The listing builds one solid part. Answer for the finished solid, in the listing's coordinates (mm). Face numbers are marked on the shaded views. A direction names the side the tool comes from. Coordinates: 2 decimals unless noted, no trailing zeros. Write each loop counter-clockwise with the first axis right and the second up, starting at its lowest first coordinate (ties: lowest second). Pieces come first, ordered by that corner, then holes. Notation, with made-up numbers: M 25.5,58 L 77.5,58 A19 ccw 77.5,63 Z; hole C 42,56.5 d7. An arc over 180 degrees is marked long. Answer as a JSON object with one key per item and string values. Group by question number.
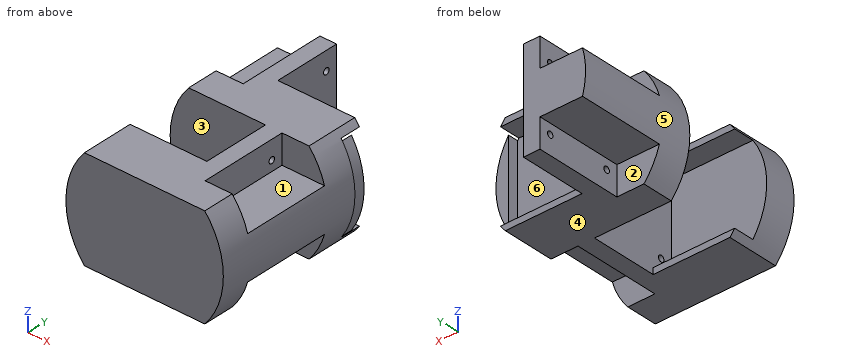
from build123d import *

# Parameters (mm, degrees)
SKETCH1_W           = 76
SKETCH1_H           = 43
BOSS_EXTRUDE1_DEPTH = 15
SKETCH3_W           = 30
SKETCH3_H           = 43
BOSS_EXTRUDE2_DEPTH = 42.1
BOSS_EXTRUDE3_START = 42.1
SKETCH4_W           = 76
SKETCH4_H           = 43
BOSS_EXTRUDE3_DEPTH = 15
SKETCH5_W           = 30
SKETCH5_H           = 43
BOSS_EXTRUDE4_DEPTH = 42.1
BOSS_EXTRUDE5_DEPTH = 3
BOSS_EXTRUDE6_DEPTH = 3
SKETCH2_OUTSIDE_W   = 107.134
SKETCH2_OUTSIDE_H   = 80.134
SKETCH2_OUTSIDE_R   = 38
CUT_EXTRUDE1_DEPTH  = 123.82463108
BOSS_EXTRUDE7_DEPTH = 5
CUT_EXTRUDE2_START  = 16
SKETCH9_W           = 14
SKETCH9_H           = 42.1
CUT_EXTRUDE2_DEPTH  = 40
CUT_EXTRUDE3_START  = -8
SKETCH10_W          = 14
SKETCH10_H          = 42.1
CUT_EXTRUDE3_DEPTH  = 40
SKETCH11_R          = 1.5
CUT_EXTRUDE4_DEPTH  = 60


with BuildPart() as part:
    # Sketch1 → Boss-Extrude1 (new body)
    with BuildSketch(Plane(origin=(0, 0, 0), x_dir=(1, 0, 0), z_dir=(0, 1, 0))):
        Rectangle(SKETCH1_W, SKETCH1_H)
    extrude(amount=BOSS_EXTRUDE1_DEPTH)

    # Sketch3 → Boss-Extrude2 (add)
    with BuildSketch(Plane(origin=(0, 15, 0), x_dir=(1, 0, 0), z_dir=(0, 1, 0))):
        with Locations((23, 0)):
            Rectangle(SKETCH3_W, SKETCH3_H)
    extrude(amount=BOSS_EXTRUDE2_DEPTH)

    # Sketch4 → Boss-Extrude3 (add)
    with BuildSketch(Plane(origin=(0, 15, 0), x_dir=(1, 0, 0), z_dir=(0, 1, 0)).offset(BOSS_EXTRUDE3_START)):
        Rectangle(SKETCH4_W, SKETCH4_H)
    extrude(amount=BOSS_EXTRUDE3_DEPTH)

    # Sketch5 → Boss-Extrude4 (add)
    with BuildSketch(Plane(origin=(0, 72.1, 0), x_dir=(1, 0, 0), z_dir=(0, 1, 0))):
        with Locations((-23, 0)):
            Rectangle(SKETCH5_W, SKETCH5_H)
    extrude(amount=BOSS_EXTRUDE4_DEPTH)

    # Sketch6 → Boss-Extrude5 (add)
    with BuildSketch(Plane.XY.offset(21.5)):
        Polygon((-38, 0), (38, 0), (38, 82.1), (-8, 82.1), (-8, 114.2), (-38, 114.2), (-38, 57.1), (8, 57.1), (8, 25), (-38, 25), align=None)
    extrude(amount=BOSS_EXTRUDE5_DEPTH)

    # Sketch7 → Boss-Extrude6 (add)
    with BuildSketch(Plane(origin=(0, 0, -21.5), x_dir=(-1, 0, 0), z_dir=(0, 0, -1))):
        Polygon((-38, 0), (38, 0), (38, 15), (38, 25), (-8, 25), (-8, 57.1), (38, 57.1), (38, 114.2), (8, 114.2), (8, 82.1), (-38, 82.1), (-38, 72.1), align=None)
    extrude(amount=BOSS_EXTRUDE6_DEPTH)

    # Sketch2 outside → Cut-Extrude1 (cut, through all)
    with BuildSketch(Plane(origin=(0, 0, 0), x_dir=(1, 0, 0), z_dir=(0, 1, 0))):
        Rectangle(SKETCH2_OUTSIDE_W, SKETCH2_OUTSIDE_H)
        Circle(SKETCH2_OUTSIDE_R, mode=Mode.SUBTRACT)
    extrude(amount=CUT_EXTRUDE1_DEPTH, mode=Mode.SUBTRACT)

    # Sketch8 → Boss-Extrude7 (add)
    with BuildSketch(Plane(origin=(0, 72.1, 0), x_dir=(1, 0, 0), z_dir=(0, 1, 0))):
        with BuildLine():
            Line((31.9, -20.64921306), (31.9, 20.64921306))
            ThreePointArc((31.9, 20.64921306), (38, 0), (31.9, -20.64921306))
        make_face()
    extrude(amount=BOSS_EXTRUDE7_DEPTH)

    # Sketch9 → Cut-Extrude2 (cut)
    with BuildSketch(Plane(origin=(0, 0, 0), x_dir=(0, 0, -1), z_dir=(1, 0, 0)).offset(CUT_EXTRUDE2_START)):
        with Locations((-17.5, 36.05)):
            Rectangle(SKETCH9_W, SKETCH9_H)
        with Locations((17.5, 36.05)):
            Rectangle(SKETCH9_W, SKETCH9_H)
    extrude(amount=CUT_EXTRUDE2_DEPTH, mode=Mode.SUBTRACT)

    # Sketch10 → Cut-Extrude3 (cut)
    with BuildSketch(Plane(origin=(-8, 0, 0), x_dir=(0, 0, -1), z_dir=(1, 0, 0)).offset(CUT_EXTRUDE3_START)):
        with Locations((-17.5, 93.15)):
            Rectangle(SKETCH10_W, SKETCH10_H)
        with Locations((17.5, 93.15)):
            Rectangle(SKETCH10_W, SKETCH10_H)
    extrude(amount=-CUT_EXTRUDE3_DEPTH, mode=Mode.SUBTRACT)

    # Sketch11 → Cut-Extrude4 (cut)
    with BuildSketch(Plane(origin=(16, 0, 0), x_dir=(0, 0, -1), z_dir=(1, 0, 0))):
        with Locations((-15.45, 20.6)):
            Circle(SKETCH11_R)
        with Locations((15.45, 20.6)):
            Circle(SKETCH11_R)
        with Locations((15.45, 51.5)):
            Circle(SKETCH11_R)
        with Locations((-15.45, 51.5)):
            Circle(SKETCH11_R)
    cut_extrude4 = extrude(amount=-CUT_EXTRUDE4_DEPTH, mode=Mode.SUBTRACT)

    # Mirror1: Cut-Extrude4 across plane
    add(cut_extrude4.mirror(Plane.ZX.offset(64.6)), mode=Mode.SUBTRACT)


solid = part.part
Item 1: A cutting plane is placed at C-C, the plane z = 15.5. State how many separate pieces and enclosed holes the cut face has, and give its area (3 significant figures).
Item 2: A tool of negligible diameter and unlimited length cuts with its end or side. For the marked faces 1, 2 and 3, from which of +Z, -Z, +X, -X, +Y, -Y can it reach the whole face along a straight path? Write none if from no direction.
Item 3: A cutting plane is placed at A-A, the plane y = 20.6. Write down the section's boundary in (x, z), and give its area (3 significant figures).
Item 4: A cutting plane is placed at D-D, the plane z = 3. Write down the section's boundary in (x, y), and give its area (3 significant figures).
Item 5: A cutting plane is placed at B-B, the plane x = -23. Write down the section's boundary in (y, z), and give its area (3 significant figures).
Item 6: For a pull along X with two mould halves and no side action, classify the marked faces 4, 5 and 6 as +X half, -X half, draft (parallel to the pull), parting line (faces both ways), or undercut.
Item 7: Consider L1, parallel to Y at x = 12.5, z = -15.45; L2, parallel to Z at x = -12, y = 77.7; L3, parallel to Y at x = 21, z = 21. Determine where each line is inside the solid, lowest interval first. Write a range as from..to.
Item 8: Flat-ended cylindrical pins translate along their axes: pin 1 Ø10 at (y, z) = (74.5, -19.5) entering from +X; pin 2 Ø5 at (y, z) = (20.6, -15.45) entering from -X; pin 3 Ø4 at (x, z) = (21.5, 17) entering from +Y. Find the tip coordinate at first contact, or state that the pin passes through.
Answer:
{
 "1": {"separate pieces": "5", "enclosed holes": "0", "area": "2,670 mm2"},
 "2": {"face 1": "+Z, +X", "face 2": "-Z, -X, +Y", "face 3": "+Z, -Z, -X"},
 "3": {"outline": "M -31.33,-21.5 A38 ccw -29.05,-24.5 L 16,-24.5 L 16,-16.95 L 8,-16.95 L 8,-21.5 Z; M -31.33,21.5 L 8,21.5 L 8,16.95 L 16,16.95 L 16,24.5 L -29.05,24.5 A38 ccw Z; M 8,-13.95 L 16,-13.95 L 16,-10.5 L 36.52,-10.5 A38 ccw 36.52,10.5 L 16,10.5 L 16,13.95 L 8,13.95 Z", "area": "1,030 mm2"},
 "4": {"outline": "M -37.88,0 L 37.88,0 L 37.88,77.1 L 31.9,77.1 L 31.9,72.1 L -8,72.1 L -8,114.2 L -37.88,114.2 L -37.88,57.1 L 8,57.1 L 8,15 L -37.88,15 Z", "area": "4,820 mm2"},
 "5": {"outline": "M 0,-24.5 L 25,-24.5 L 25,-21.5 L 15,-21.5 L 15,21.5 L 25,21.5 L 25,24.5 L 0,24.5 Z; M 57.1,-24.5 L 72.1,-24.5 L 72.1,-10.5 L 114.2,-10.5 L 114.2,10.5 L 72.1,10.5 L 72.1,24.5 L 57.1,24.5 Z", "area": "2,410 mm2"},
 "6": {"face 4": "draft", "face 5": "-X half", "face 6": "undercut"},
 "7": {"L1": "0..19.1, 22.1..50, 53..72.1", "L2": "-24.5..-16.95, -13.95..13.95, 16.95..24.5", "L3": "0..15, 57.1..72.1"},
 "8": {"pin 1": "x = 35.12", "pin 2": "x = 8", "pin 3": "y = 72.1"}
}
